from build123d import *

# Parameters (mm, degrees)
BOSS_EXTRUDE1_DEPTH = 0.5
SKETCH2_W           = 3
SKETCH2_H           = 1
BOSS_EXTRUDE2_DEPTH = 1.5
SKETCH3_W           = 0.4
SKETCH3_H           = 4
BOSS_EXTRUDE3_DEPTH = 1


with BuildPart() as part:
    # Sketch1 → Boss-Extrude1 (new body)
    with BuildSketch(Plane.XY):
        with BuildLine():
            Line((-4.5, -7.5), (4.5, -7.5))
            ThreePointArc((4.5, -7.5), (5.207106781, -7.207106781), (5.5, -6.5))
            Line((5.5, -6.5), (5.5, 6.5))
            ThreePointArc((5.5, 6.5), (5.207106781, 7.207106781), (4.5, 7.5))
            Line((4.5, 7.5), (-4.5, 7.5))
            ThreePointArc((-4.5, 7.5), (-5.207106781, 7.207106781), (-5.5, 6.5))
            Line((-5.5, 6.5), (-5.5, -6.5))
            ThreePointArc((-5.5, -6.5), (-5.207106781, -7.207106781), (-4.5, -7.5))
        make_face()
    extrude(amount=BOSS_EXTRUDE1_DEPTH)

    # Sketch2 → Boss-Extrude2 (add)
    with BuildSketch(Plane.XY.offset(0.5)):
        with Locations((0, 7)):
            Rectangle(SKETCH2_W, SKETCH2_H)
    extrude(amount=BOSS_EXTRUDE2_DEPTH)

    # Sketch3 → Boss-Extrude3 (add)
    with BuildSketch(Plane.XY.offset(0.5)):
        with Locations((-4.7, 0)):
            Rectangle(SKETCH3_W, SKETCH3_H)
    boss_extrude3 = extrude(amount=BOSS_EXTRUDE3_DEPTH)

    # Mirror2: Boss-Extrude3 across plane
    add(boss_extrude3.mirror(Plane(origin=(0, 0, 0), x_dir=(0, 0, 1), z_dir=(1, 0, 0))))


solid = part.part
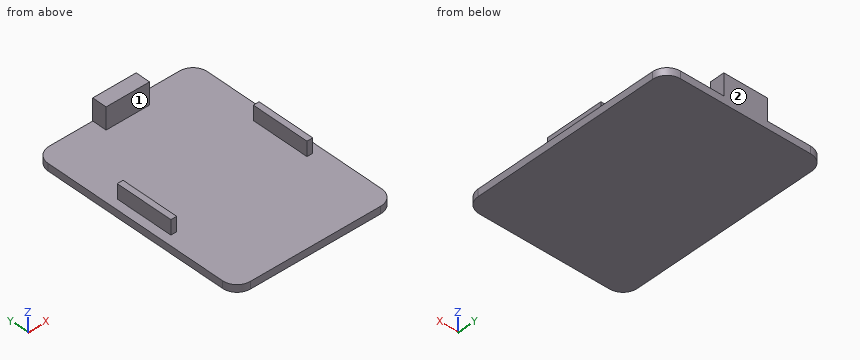
Input: part model. Units: mm. Frame: model coordinates. Face numbers are marked on the shaded views. A direction names the side the tool comes from. Coordinates: 2 decimals unless noted, no trailing zeros. Loops run counter-clockwise (first coordinate to the right, second up) from the corner with the lowest first, then second, coordinate; pieces in that order, holes last. Notation, with made-up numbers: (78, -20) -> (133, -20) arc R13 cw to (133, -1) -> close; hole circle Ø3 at (5.5, -36). An arc over 180 degrees is marked (long way). One line per item, written item: value.
(1) Cut plane B-B (y = 1). Output: boundary loops of the cut face in (x, z).
Answer below:
outline: (-5.5, 0) -> (5.5, 0) -> (5.5, 0.5) -> (4.9, 0.5) -> (4.9, 1.5) -> (4.5, 1.5) -> (4.5, 0.5) -> (-4.5, 0.5) -> (-4.5, 1.5) -> (-4.9, 1.5) -> (-4.9, 0.5) -> (-5.5, 0.5) -> close
(2) Ray query, line 1 along X through (y, z) = (-0.5, 1.25); line 2 along Y through (x, z) = (1, 1.55); line 3 along Z through (x, y) = (2.25, -6.5). Return the intervals inside material, ascending.
Answer below:
line 1: x = -4.9 to -4.5, 4.5 to 4.9
line 2: y = 6.5 to 7.5
line 3: z = 0 to 0.5
(3) Cut plane A-A (z = 0.8). Output: boundary loops of the cut face in (x, y), then the cut area to 3 significant figures.
Answer below:
outline: (-4.9, -2) -> (-4.5, -2) -> (-4.5, 2) -> (-4.9, 2) -> close; (-1.5, 6.5) -> (1.5, 6.5) -> (1.5, 7.5) -> (-1.5, 7.5) -> close; (4.5, -2) -> (4.9, -2) -> (4.9, 2) -> (4.5, 2) -> close
area: 6.20 mm2
(4) Pin query (flat end, axial travel): pin 1 Ø1 at (x, y) = (-4, 3) entering from +Z; pin 2 Ø0.8 at (y, z) = (0.5, 1) entering from +X; pin 3 Ø1.5 at (x, y) = (-4.5, 0.5) entering from +Z. Return the tip coordinate at first contact, or that it passes through.
Answer below:
pin 1: stops at z = 0.5
pin 2: stops at x = 4.9
pin 3: stops at z = 1.5
(5) Set-up query: the marked faces 1 and 2. Return all of +Z, -Z, +X, -X, +Y, -Y with unobstructed straight access to the full face (end or side cutting, diameter ignored); none if empty.
Answer below:
face 1: +Z, +X, -X, -Y
face 2: +Z, -Z, +X, -X, +Y
(6) Cut plane C-C (x = -0.5). Output: boundary loops of the cut face in (y, z), then the cut area to 3 significant figures.
Answer below:
outline: (-7.5, 0) -> (7.5, 0) -> (7.5, 2) -> (6.5, 2) -> (6.5, 0.5) -> (-7.5, 0.5) -> close
area: 9.00 mm2
(7) Cut plane D-D (x = -3.75). Output: boundary loops of the cut face in (y, z), then the cut area to 3 significant figures.
Answer below:
outline: (-7.5, 0) -> (7.5, 0) -> (7.5, 0.5) -> (-7.5, 0.5) -> close
area: 7.50 mm2
